Check sheet for the modelled part. Datum: model origin and axes. Units: mm. A direction names the side the tool comes from. Coordinates: 2 decimals unless noted, no trailing zeros. Order: outer loops, then holes, each group sorted by start corner. A loop starts at its lowest first (then second) coordinate and runs counter-clockwise, first axis right, second up.
1. Cross-section at C-C (z = 11.25). Enter the section's corners in (x, y).
2. Set-up check for faces 1 (the flat face through (-1, 0, 12.5)), 2 (the flat face through (0, 0, 0)): record each of +Z, -Z, +X, -X, +Y, -Y from which the full face is reachable in a straight line by a thin tool's end or side.
3. Thickness scan on line 1 (Z direction, x = 0.8, y = 1); line 2 (X direction, y = 0.1, z = 5); line 3 (Y direction, x = 0, z = 14). Record the ranges inside material, lowest first.
4. Gauge pin test, flat ends, axial feed: pin 1 Ø3 at (y, z) = (-1.5, 13) entering from +X; pin 2 Ø1.5 at (x, z) = (0.5, 10.5) entering from +Y. Record the tip position at first contact, or that the pin passes through.
5. Cross-section at A-A (x = 0). Enter the section's corners in (y, z).
```python
from build123d import *

# Parameters (mm, degrees)
SKETCH_R     = 2.5
PAD_DEPTH    = 2
FILLET_R     = 1
SKETCH001_R  = 1.5
PAD001_DEPTH = 10.5
SKETCH002_R  = 0.75
PAD002_DEPTH = 3


with BuildPart() as part:
    # Sketch → Pad (new body)
    with BuildSketch(Plane.XY):
        Circle(SKETCH_R)
    extrude(amount=PAD_DEPTH)

    # Fillet
    fillet_edges = [part.edges().sort_by_distance(p)[0] for p in [
        (-2.5, 0, 0),
    ]]
    fillet(fillet_edges, radius=FILLET_R)

    # Sketch001 (on DatumPlane) → Pad001 (join)
    with BuildSketch(Plane.XY.offset(2)):
        Circle(SKETCH001_R)
    extrude(amount=PAD001_DEPTH)

    # Sketch002 (on DatumPlane) → Pad002 (join)
    with BuildSketch(Plane.XY.offset(12.5)):
        Circle(SKETCH002_R)
    extrude(amount=PAD002_DEPTH)


solid = part.part
```
Data:
1. outline: circle Ø3 at (0, 0)
2. face 1: +Z
2. face 2: -Z, +X, -X, +Y, -Y
3. line 1: z = 0 to 12.5
3. line 2: x = -1.5 to 1.5
3. line 3: y = -0.75 to 0.75
4. pin 1: stops at x = 1.5
4. pin 2: stops at y = 1.5
5. outline: (-2.5, 1) arc R1 ccw to (-1.5, 0) - (1.5, 0) arc R1 ccw to (2.5, 1) - (2.5, 2) - (1.5, 2) - (1.5, 12.5) - (0.75, 12.5) - (0.75, 15.5) - (-0.75, 15.5) - (-0.75, 12.5) - (-1.5, 12.5) - (-1.5, 2) - (-2.5, 2) - close
